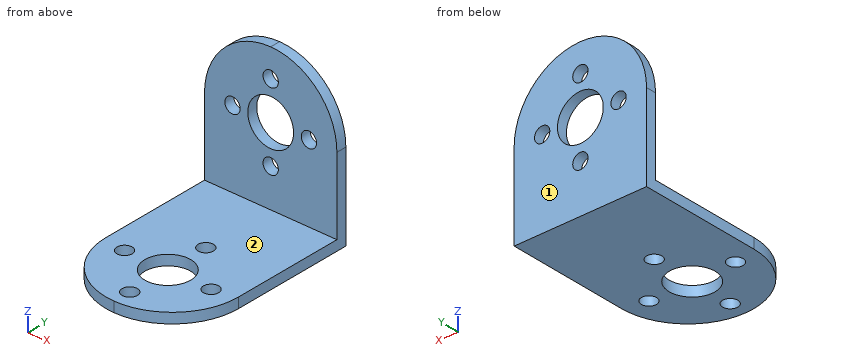
from build123d import *

# Parameters (mm, degrees)
BOSS_EXTRUDE1_DEPTH = 26
SKETCH4_R           = 4.5
SKETCH4_R_2         = 1.5
CUT_EXTRUDE2_DEPTH  = 3
SKETCH5_R           = 1.5
SKETCH5_R_2         = 4.5
CUT_EXTRUDE3_DEPTH  = 3


with BuildPart() as part:
    # Sketch2 → Boss-Extrude1 (new body)
    with BuildSketch(Plane(origin=(0, 0, 0), x_dir=(0, 0, -1), z_dir=(1, 0, 0))):
        Polygon((-15.5, 1), (14.5, 1), (14.5, -36), (12.5, -36), (12.5, -1), (-15.5, -1), align=None)
    extrude(amount=BOSS_EXTRUDE1_DEPTH)

    # Sketch4 → Cut-Extrude2 (cut, through all)
    with BuildSketch(Plane.XY.offset(-12.5)):
        with Locations((13, -24)):
            Circle(SKETCH4_R)
        with Locations((4.5, -24)):
            Circle(SKETCH4_R_2)
        with Locations((13, -32.5)):
            Circle(SKETCH4_R_2)
        with Locations((21.5, -24)):
            Circle(SKETCH4_R_2)
        with Locations((13, -15.5)):
            Circle(SKETCH4_R_2)
        with BuildLine():
            ThreePointArc((13, -36), (3.807611845, -32.192388155), (0, -23))
            Line((0, -23), (0, -36))
            Line((0, -36), (13, -36))
        make_face()
        with BuildLine():
            ThreePointArc((26, -23), (22.192388155, -32.192388155), (13, -36))
            Line((13, -36), (26, -36))
            Line((26, -36), (26, -23))
        make_face()
    extrude(amount=-CUT_EXTRUDE2_DEPTH, mode=Mode.SUBTRACT)

    # Sketch5 → Cut-Extrude3 (cut, through all)
    with BuildSketch(Plane.XZ.offset(1)):
        with Locations((5.5, 2.5)):
            Circle(SKETCH5_R)
        with Locations((13, -5)):
            Circle(SKETCH5_R)
        with Locations((13, 2.5)):
            Circle(SKETCH5_R_2)
        with Locations((20.5, 2.5)):
            Circle(SKETCH5_R)
        with BuildLine():
            Line((13, 15.5), (0, 15.5))
            Line((0, 15.5), (0, 2.5))
            ThreePointArc((0, 2.5), (3.807611845, 11.692388155), (13, 15.5))
        make_face()
        with BuildLine():
            Line((26, 15.5), (13, 15.5))
            ThreePointArc((13, 15.5), (22.192388155, 11.692388155), (26, 2.5))
            Line((26, 2.5), (26, 15.5))
        make_face()
        with Locations((13, 10)):
            Circle(SKETCH5_R)
    extrude(amount=-CUT_EXTRUDE3_DEPTH, mode=Mode.SUBTRACT)


solid = part.part
Read the model definition and answer for the solid it produces. Units are mm, in the model's axes. Face numbers are marked on the shaded views. A direction names the side the tool comes from. Coordinates: 2 decimals unless noted, no trailing zeros. Order: outer loops, then holes, each group sorted by start corner. A loop starts at its lowest first (then second) coordinate and runs counter-clockwise, first axis right, second up. Notation, with made-up numbers: (82.25, 41) -> (95.25, 41) arc R27 ccw to (95.25, 76) -> close; hole circle Ø6 at (1, -34). An arc over 180 degrees is marked (long way). Answer as a JSON object with one key per item and string values.
1) Each of these flat-tipped pins is pushed along its axis until it touches: pin 1 (3 mm diameter, centred on x = 12.5, y = -29.5, fed in from +Z); pin 2 (4 mm diameter, centred on x = 5.5, z = 2.5, fed in from -Y); pin 3 (1.8 mm diameter, centred on x = 20.5, z = 2.5, fed in from -Y); pin 4 (10 mm diameter, centred on y = -5.5, z = 8, fed in from -X). Where does it stop, or does it pass through?
Model answer:
{"pin 1": "stops at z = -12.5", "pin 2": "stops at y = -1", "pin 3": "passes through", "pin 4": "stops at x = 0.43"}
2) Consider line 1 along Y through (x, z) = (13, -13.3); line 2 along Z through (x, y) = (13, -0.1); line 3 along Z through (x, y) = (3.75, -1.5). Determine where each line is inside the solid, lowest interval first. Write a range as from..to.
Model answer:
{"line 1": "y = -36..-34, -31..-28.5, -19.5..-17, -14..1", "line 2": "z = -14.5..-6.5, -3.5..-2, 7..8.5, 11.5..15.5", "line 3": "z = -14.5..-12.5"}
3) A cutting plane is placed at C-C, the plane x = 4.5. Determine the outline of the cut face in (y, z), plus the area to 3 significant figures.
Model answer:
{"outline": "(-32.84, -14.5) -> (-25.5, -14.5) -> (-25.5, -12.5) -> (-32.84, -12.5) -> close; (-22.5, -14.5) -> (1, -14.5) -> (1, 1.38) -> (-1, 1.38) -> (-1, -12.5) -> (-22.5, -12.5) -> close; (-1, 3.62) -> (1, 3.62) -> (1, 12.34) -> (-1, 12.34) -> close", "area": "107 mm²"}
4) A tool of negligible diameter and unlimited length cuts with its end or side. For the marked faces 1 and 2, from which of +Z, -Z, +X, -X, +Y, -Y can it reach the whole face along a straight path? Write none if from no direction.
Model answer:
{"face 1": "+Z, -Z, +X, -X, +Y", "face 2": "+Z, +X, -X, -Y"}
5) A cutting plane is placed at A-A, the plane y = -15.5. Determine the outline of the cut face in (x, z).
Model answer:
{"outline": "(0, -14.5) -> (11.5, -14.5) -> (11.5, -12.5) -> (0, -12.5) -> close; (14.5, -14.5) -> (26, -14.5) -> (26, -12.5) -> (14.5, -12.5) -> close"}
6) A cutting plane is placed at B-B, the plane z = -5. Determine the outline of the cut face in (x, y), plus the area to 3 significant figures.
Model answer:
{"outline": "(0, -1) -> (11.5, -1) -> (11.5, 1) -> (0, 1) -> close; (14.5, -1) -> (26, -1) -> (26, 1) -> (14.5, 1) -> close", "area": "46.0 mm²"}
7) A cutting plane is placed at D-D, the plane y = -24. Determine the outline of the cut face in (x, z).
Model answer:
{"outline": "(0.04, -14.5) -> (3, -14.5) -> (3, -12.5) -> (0.04, -12.5) -> close; (6, -14.5) -> (8.5, -14.5) -> (8.5, -12.5) -> (6, -12.5) -> close; (17.5, -14.5) -> (20, -14.5) -> (20, -12.5) -> (17.5, -12.5) -> close; (23, -14.5) -> (25.96, -14.5) -> (25.96, -12.5) -> (23, -12.5) -> close"}
